Input: part model. Units: mm. Frame: model coordinates. Face numbers are marked on the shaded views. A direction names the side the tool comes from. Coordinates: 2 decimals unless noted, no trailing zeros. Loops run counter-clockwise (first coordinate to the right, second up) from the corner with the lowest first, then second, coordinate; pieces in that order, holes last.
Item 1: Pull-direction query (X, two-part tool) for the marked faces 3, 4 and 5; classes: released by +X, released by -X, zero draft, split by the parting line, or undercut.
Item 2: Section C-C on y = 4.5. Return loops of the section in (x, z), and give its area (3 significant figures).
Item 3: Reachability of the marked faces 1 and 2 from +Z, -Z, +X, -X, +Y, -Y: full face, straight path, thin tool, end or side. Return the list, or none.
Item 4: Section D-D on x = 2.25. Return loops of the section in (y, z).
Item 5: Ray query, line 1 along Y through (x, z) = (0, 16.25); line 2 along Y through (x, z) = (0, 7); line 3 along X through (y, z) = (1, 4.5). Return the intervals inside material, ascending.
Item 6: Contact query for flat-ended pins moving along their axis: P1, Ø3, axis at x = -4.5, z = 7, coming from the +Y side; P2, Ø3, axis at x = 2, y = -12.5, coming from the +Z side; P3, Ø1.5, axis at y = -12.5, z = 13, coming from the -X side. Output: stop coordinate, or through.
Item 7: Section B-B on z = 10. Return loops of the section in (x, y), and give its area (3 significant figures).
Item 8: Section A-A on x = 0. Return loops of the section in (y, z), and give its area (3 significant figures).
```python
from build123d import *

# Parameters (mm, degrees)
EXTRUDE_1_DEPTH     = 20
SKETCH_3_R          = 5
CUT_EXTRUDE_1_DEPTH = 25.494897428
SKETCH_5_R          = 4
EXTRUDE_2_DEPTH     = 10


with BuildPart() as part:
    # ｽｹｯﾁ2 → ﾎﾞｽ - 押し出し1 (new body)
    with BuildSketch(Plane.XY):
        with BuildLine():
            Line((-10, 0), (-10, -7.5))
            Line((-10, -7.5), (10, -7.5))
            Line((10, -7.5), (10, 0))
            ThreePointArc((10, 0), (0, 10), (-10, 0))
        make_face()
    extrude(amount=EXTRUDE_1_DEPTH)

    # ｽｹｯﾁ3 → ｶｯﾄ - 押し出し1 (cut, through all)
    with BuildSketch(Plane.XY.offset(20)):
        Circle(SKETCH_3_R)
    extrude(amount=-CUT_EXTRUDE_1_DEPTH, mode=Mode.SUBTRACT)

    # ｽｹｯﾁ5 → ﾎﾞｽ - 押し出し2 (add)
    with BuildSketch(Plane(origin=(0, -7.5, 0), x_dir=(-1, 0, 0), z_dir=(0, -1, 0))):
        with Locations(Location((0, -10, 0), (0, 0, 90))):
            Circle(SKETCH_5_R)
    extrude(amount=EXTRUDE_2_DEPTH)


solid = part.part
```
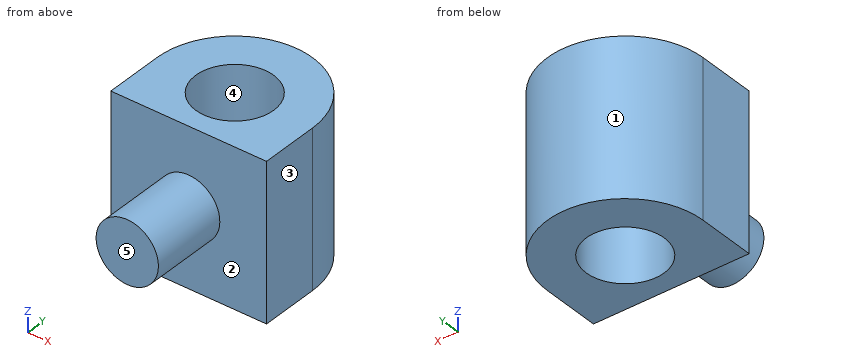
Results found:
1. face 3: released by +X
1. face 4: undercut
1. face 5: zero draft
2. outline: (-8.93, 0) - (-2.18, 0) - (-2.18, 20) - (-8.93, 20) - close; (2.18, 0) - (8.93, 0) - (8.93, 20) - (2.18, 20) - close
2. area: 270 mm2
3. face 1: +Z, -Z, +Y
3. face 2: -Y
4. outline: (-17.5, 6.69) - (-7.5, 6.69) - (-7.5, 0) - (-4.47, 0) - (-4.47, 20) - (-7.5, 20) - (-7.5, 13.31) - (-17.5, 13.31) - close; (4.47, 0) - (9.74, 0) - (9.74, 20) - (4.47, 20) - close
5. line 1: y = -7.5 to -5, 5 to 10
5. line 2: y = -17.5 to -5, 5 to 10
5. line 3: x = -9.95 to -4.9, 4.9 to 9.95
6. P1: stops at y = 9.54
6. P2: stops at z = 13.97
6. P3: stops at x = -3.31
7. outline: (-10, -7.5) - (-4, -7.5) - (-4, -17.5) - (4, -17.5) - (4, -7.5) - (10, -7.5) - (10, 0) arc R10 ccw to (-10, 0) - close; hole circle Ø10 at (0, 0)
7. area: 309 mm2
8. outline: (-17.5, 6) - (-7.5, 6) - (-7.5, 0) - (-5, 0) - (-5, 20) - (-7.5, 20) - (-7.5, 14) - (-17.5, 14) - close; (5, 0) - (10, 0) - (10, 20) - (5, 20) - close
8. area: 230 mm2
